Check sheet for the modelled part. Datum: model origin and axes. Units: mm. Face numbers are marked on the shaded views. A direction names the side the tool comes from. Coordinates: 2 decimals unless noted, no trailing zeros. Loops run counter-clockwise (first coordinate to the right, second up) from the corner with the lowest first, then second, coordinate; pieces in that order, holes last. Notation, with made-up numbers: (14, -21) - (55, -21) arc R20 ccw to (55, -8) - close; hole circle Ø2 at (82.5, 51). An arc over 180 degrees is marked (long way). Answer as a JSON object with one key per item and string values. Group by question number.
from build123d import *

# Parameters (mm, degrees)
SKETCH1_W       = 27
SKETCH1_H       = 14
HOUSING_DEPTH   = 8
WIRE_STUB_START = -23.5
SKETCH2_R       = 1.5
WIRE_STUB_DEPTH = 10


with BuildPart() as part:
    # Sketch1 → Housing (new body)
    with BuildSketch(Plane(origin=(0, 0, 0), x_dir=(1, 0, 0), z_dir=(0, 1, 0))):
        Rectangle(SKETCH1_W, SKETCH1_H)
    extrude(amount=HOUSING_DEPTH)

    # Sketch2 → Wire_Stub (add)
    with BuildSketch(Plane(origin=(0, 0, 0), x_dir=(0, 0, -1), z_dir=(1, 0, 0)).offset(WIRE_STUB_START)):
        with Locations((0, 4)):
            Circle(SKETCH2_R)
    extrude(amount=WIRE_STUB_DEPTH)


solid = part.part
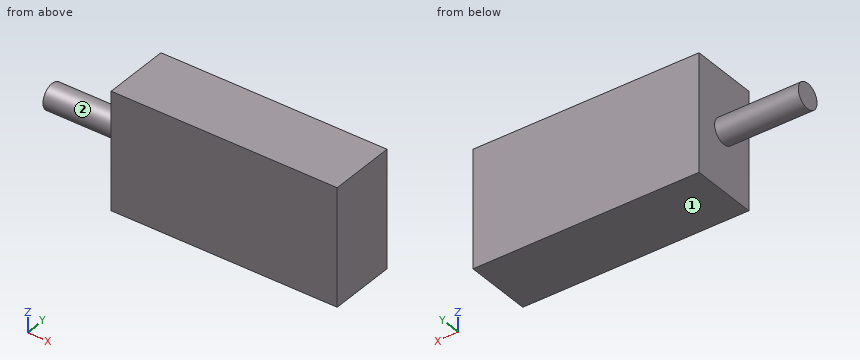
1. Gauge pin test, flat ends, axial feed: pin 1 (1.5 mm diameter, centred on x = -17.5, y = 5.5, fed in from -Z); pin 2 (3 mm diameter, centred on y = 1.5, z = 5.5, fed in from -X). Record the tip position at first contact, or that the pin passes through.
2. Sectioned sample at D-D on y = 6.75. Record the cut outline in (x, z), plus the area to 3 significant figures.
3. Material ranges on line 1 (X direction, y = 5.75, z = -4.5); line 2 (Z direction, x = -17.5, y = 3.25); line 3 (Y direction, x = -15.5, z = 1), recorded low to high.
4. Sectioned sample at A-A on z = 0. Record the cut outline in (x, y), plus the area to 3 significant figures.
5. Sectioned sample at C-C on x = -17. Record the cut outline in (y, z), plus the area to 3 significant figures.
6. Sectioned sample at B-B on y = 4. Record the cut outline in (x, z).
7. Access from +Z, -Z, +X, -X, +Y, -Y to the whole of each face (thin tool, end or side, straight path). Record for the marked faces 1 and 2.
Answers follow:
{
 "1": {"pin 1": "stops at z = -1.3", "pin 2": "stops at x = -13.5"},
 "2": {"outline": "(-13.5, -7) - (13.5, -7) - (13.5, 7) - (-13.5, 7) - close", "area": "378 mm^2"},
 "3": {"line 1": "x = -13.5 to 13.5", "line 2": "z = -1.3 to 1.3", "line 3": "y = 2.88 to 5.12"},
 "4": {"outline": "(-23.5, 2.5) - (-13.5, 2.5) - (-13.5, 0) - (13.5, 0) - (13.5, 8) - (-13.5, 8) - (-13.5, 5.5) - (-23.5, 5.5) - close", "area": "246 mm^2"},
 "5": {"outline": "circle Ø3 at (4, 0)", "area": "7.07 mm^2"},
 "6": {"outline": "(-23.5, -1.5) - (-13.5, -1.5) - (-13.5, -7) - (13.5, -7) - (13.5, 7) - (-13.5, 7) - (-13.5, 1.5) - (-23.5, 1.5) - close"},
 "7": {"face 1": "-Z, +X, -X, +Y, -Y", "face 2": "-X"}
}
